```python
from build123d import *

# Parameters (mm, degrees)
RESSALTO_EXTRUS_O1_DEPTH = 12
FILETE1_START            = -1
FILETE1_DEPTH            = 5.566394674
FILETE1_2_DEPTH          = 0.5


with BuildPart() as part:
    # Esboço1 → Ressalto-extrusão1 (new body)
    with BuildSketch(Plane.XY):
        Polygon((0, 0), (60, 0), (60, 0.5), (0.309409388, 0.5), (-4.01451095, 9.172442523), (-4.461978131, 8.949343616), align=None)
    extrude(amount=RESSALTO_EXTRUS_O1_DEPTH)

    # Filete1: read off the stored shape, not the designer's step
    # Filete1 outline → Filete1 (cut)
    with BuildSketch(Plane(origin=(0, 0, 0), x_dir=(1, 0, 0), z_dir=(0, 1, 0)).offset(FILETE1_START)):
        with BuildLine():
            Line((60, -12), (60, -6))
            add(Edge.make_bspline(
                [(54, -12), (60, -12), (60, -6)],
                knots=[0, 0, 0, 1, 1, 1], degree=2, weights=[1, 0.707106781, 1]))
            Line((54, -12), (60, -12))
        make_face()
        with BuildLine():
            add(Edge.make_bspline(
                [(60, -6), (60, 0), (54, 0)],
                knots=[0, 0, 0, 1, 1, 1], degree=2, weights=[1, 0.707106781, 1]))
            Line((60, -6), (60, 0))
            Line((60, 0), (54, 0))
        make_face()
    extrude(amount=FILETE1_DEPTH, mode=Mode.SUBTRACT)

    # Filete1 2 outline → Filete1 2 (cut)
    with BuildSketch(Plane(origin=(0, 0, 0), x_dir=(0.44619781310978035, -0.8949343616020392, 0), z_dir=(0.8949343616020393, 0.44619781310977996, 0))):
        with BuildLine():
            Line((-10, 0), (-10, -6))
            add(Edge.make_bspline(
                [(-10, -6), (-10, 0), (-4, 0)],
                knots=[0, 0, 0, 1, 1, 1], degree=2, weights=[1, 0.707106781, 1]))
            Line((-4, 0), (-10, 0))
        make_face()
        with BuildLine():
            add(Edge.make_bspline(
                [(-4, -12), (-10, -12), (-10, -6)],
                knots=[0, 0, 0, 1, 1, 1], degree=2, weights=[1, 0.707106781, 1]))
            Line((-10, -6), (-10, -12))
            Line((-10, -12), (-4, -12))
        make_face()
    extrude(amount=FILETE1_2_DEPTH, mode=Mode.SUBTRACT)


solid = part.part
```
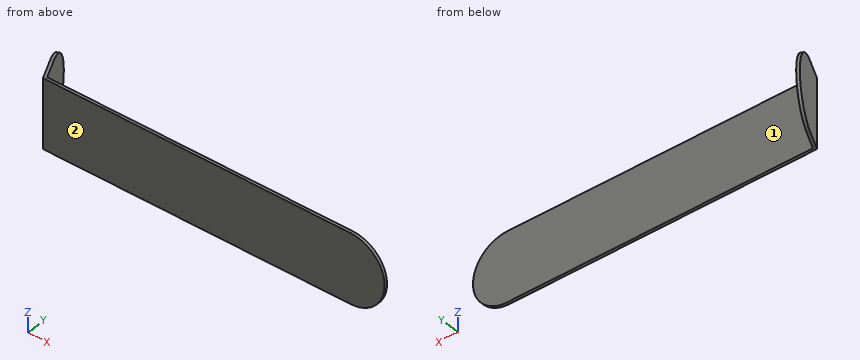
Input: part model. Units: mm. Frame: model coordinates. Face numbers are marked on the shaded views. A direction names the side the tool comes from. Coordinates: 2 decimals unless noted, no trailing zeros. Write each loop counter-clockwise with the first axis right and the second up, starting at its lowest first coordinate (ties: lowest second). Pieces come first, ordered by that corner, then holes. Notation, with made-up numbers: (22.5, 79) -> (48.5, 79) arc R23 ccw to (48.5, 110) -> close; hole circle Ø8 at (77.25, 21). An arc over 180 degrees is marked (long way). Write each question's results on one line, items separated by ' | '.
Item 1: Material intervals for probe 1 along Y at (x, z) = (54, 10.75); probe 2 along X at (y, z) = (4.75, 2); probe 3 along X at (y, z) = (4, 2.5), sorted ascending.
Conclusion:
probe 1: y = 0 to 0.5 | probe 2: x = -2.37 to -1.81 | probe 3: x = -1.99 to -1.44
Item 2: Pin query (flat end, axial travel): pin 1 Ø3.5 at (x, z) = (45, 9) entering from +Y. Return the tip coordinate at first contact, or that it passes through.
Conclusion:
pin 1: stops at y = 0.5
Item 3: Set-up query: the marked faces 1 and 2. Return all of +Z, -Z, +X, -X, +Y, -Y with unobstructed straight access to the full face (end or side cutting, diameter ignored); none if empty.
Conclusion:
face 1: +Z, -Z, +X, +Y | face 2: +Z, -Z, +X, -X, -Y
Item 4: Section query A-A on x = 8.5. Return loops of the section in (y, z).
Conclusion:
outline: (0, 0) -> (0.5, 0) -> (0.5, 12) -> (0, 12) -> close
Item 5: Section query B-B on y = 2. Return loops of the section in (x, z).
Conclusion:
outline: (-1, 0) -> (-0.44, 0) -> (-0.44, 12) -> (-1, 12) -> close
